Part model, mm, in its own coordinate system. A direction names the side the tool comes from. Round coordinates to 2 decimals unless told otherwise and drop trailing zeros. Write each loop counter-clockwise with the first axis right and the second up, starting at its lowest first coordinate (ties: lowest second). Pieces come first, ordered by that corner, then holes. Notation, with made-up numbers: (-35, 4.25) -> (-25, 4.25) arc R16 ccw to (-25, 12.25) -> close; hole circle Ø9 at (-8, 0.5). An arc over 180 degrees is marked (long way). Use CSV: the item, a comma, the result in double quotes. Start each with the question number.
(1) Which spindle directions (+Z, -Z, +X, -X, +Y, -Y) get a long thin tool onto all of the face, cutting with end or side? Do faces 1 (the flat face through (0, 25, 5)), 2 (the flat face through (0, 0, 10)). Say none if no direction does.
(2) Two-plate mould, pull along X, no slides. Class faces 3 (the flat face through (-9.34, 24.65, 12.68)), 4 (the flat face through (9.43, 24.65, 12.32)), 5 (the flat face through (0, 25, 0)), 6 (the cylindrical face through (-0.521, 28.966, 15.14)): released by +X, released by -X, zero draft, split by the parting line, or undercut.
(3) Probe line 1 (Y direction, x = 0, z = 15.5); line 2 (Y direction, x = 1, z = 21); line 3 (X direction, y = 31, z = 4.5). List the from-to ranges inside material, lowest first. Write a range as [from, to].
(4) Saw through at D-D (z = 6). Give the cut face in (x, y).
(5) Saw through at C-C (z = 14). Give the cut face in (x, y).
(6) Drop flat-ended pins along their axis: pin 1 (6 mm diameter, centred on y = 35, z = 22.5, fed in from -X); pin 2 (10 mm diameter, centred on y = 32, z = 16, fed in from +X); pin 3 (6.5 mm diameter, centred on x = 0, y = 25, fed in from +Z). Give the stop position or say it passes through.
(7) Saw through at A-A (y = 25). Give the cut face in (x, z), plus the area to 3 significant figures.
(8) Saw through at B-B (x = 0). Give the cut face in (y, z).
```python
from build123d import *

# Parameters (mm, degrees)
F1_DEPTH = 50
F2_R     = 4
F3_DEPTH = 20


with BuildPart() as f1:
    # F0 (on Front) → F1 (new body)
    with BuildSketch(Plane.XZ):
        Polygon((-6.2668, 25), (-12.5, 0), (12.5, 0), (6.2668, 25), align=None)
    extrude(amount=-F1_DEPTH)

    # F2 (on face) → F3 (cut)
    with BuildSketch(Plane.XY.offset(25)):
        with Locations((0, 25)):
            Circle(F2_R)
    extrude(amount=-F3_DEPTH, mode=Mode.SUBTRACT)


solid = f1.part
```
Answers:
1,face 1,"+Z"
1,face 2,"+Z, -Z, +X, -X, -Y"
2,face 3,"released by -X"
2,face 4,"released by +X"
2,face 5,"zero draft"
2,face 6,"undercut"
3,line 1,"y = [0, 21], [29, 50]"
3,line 2,"y = [0, 21.13], [28.87, 50]"
3,line 3,"x = [-11.38, 11.38]"
4,outline,"(-11, 0) -> (11, 0) -> (11, 50) -> (-11, 50) -> close; hole circle Ø8 at (0, 25)"
5,outline,"(-9.01, 0) -> (9.01, 0) -> (9.01, 50) -> (-9.01, 50) -> close; hole circle Ø8 at (0, 25)"
6,pin 1,"stops at x = -7.64"
6,pin 2,"stops at x = 9.76"
6,pin 3,"stops at z = 5"
7,outline,"(-12.5, 0) -> (12.5, 0) -> (6.27, 25) -> (4, 25) -> (4, 5) -> (-4, 5) -> (-4, 25) -> (-6.27, 25) -> close"
7,area,"309 mm²"
8,outline,"(0, 0) -> (50, 0) -> (50, 25) -> (29, 25) -> (29, 5) -> (21, 5) -> (21, 25) -> (0, 25) -> close"
